Source: CAD feature listing. Evaluate the final solid. Frame: model axes, mm. Give positions to 0.01 mm unless a question says otherwise; leave off trailing zeros. Write each loop counter-clockwise with the first axis right and the second up, starting at its lowest first coordinate (ties: lowest second). Pieces come first, ordered by that corner, then holes.
```python
from build123d import *

# Parameters (mm, degrees)
BOSS_EXTRUDE1_DEPTH = 5


with BuildPart() as part:
    # Sketch1 → Boss-Extrude1 (new body)
    with BuildSketch(Plane.XY):
        Polygon((170, -430), (210, -430), (210, -435), (240, -435), (240, -430), (280, -430), (280, -435), (310, -435), (310, -430), (350, -430), (350, -435), (380, -435), (380, -430), (440.000271395, -430), (445, -430), (445, -422.5), (440.000271395, -422.5), (440.000271395, -407.5), (445, -407.5), (445, -400), (440.000271395, -400), (9.999728605, -400), (5, -400), (5, -407.5), (9.999728605, -407.5), (9.999728605, -422.5), (5, -422.5), (5, -430), (9.999728605, -430), (70, -430), (70, -435), (100, -435), (100, -430), (140, -430), (140, -435), (170, -435), align=None)
    extrude(amount=-BOSS_EXTRUDE1_DEPTH)


solid = part.part
```
1. Section query C-C (y = -416). Return loops of the section in (x, z), plus the area to 3 significant figures.
2. Line query: probe 1 along X at (y, z) = (-431, -1.9); probe 2 along Y at (x, z) = (398, -3.3); probe 3 along X at (y, z) = (-422, -3.35). Output: solid intervals per line, ascending.
3. Section query B-B (x = 334.5). Return loops of the section in (y, z), plus the area to 3 significant figures.
4. Pin query (flat end, axial travel): P1, Ø1.5, axis at x = 8.5, z = -3.5, coming from the -Y side; P2, Ø1.5, axis at y = -418.5, z = -4, coming from the +X side; P3, Ø2.5, axis at y = -432.5, z = -3.5, coming from the +X side. Return the tip coordinate at first contact, or that it passes through.
The answers:
1. outline: (10, -5) - (440, -5) - (440, 0) - (10, 0) - close
1. area: 2,150 mm2
2. probe 1: x = 70 to 100, 140 to 170, 210 to 240, 280 to 310, 350 to 380
2. probe 2: y = -430 to -400
2. probe 3: x = 10 to 440
3. outline: (-430, -5) - (-400, -5) - (-400, 0) - (-430, 0) - close
3. area: 150 mm2
4. P1: stops at y = -430
4. P2: stops at x = 440
4. P3: stops at x = 380
